from build123d import *

# Parameters (mm, degrees)
F0_R        = 10.9982
F0_R_2      = 11
F1_DEPTH    = 7
F2_T1_DEPTH = 57
F2_T4_ANGLE = 180
F2_T6_ANGLE = 180


# Not quite as in the source:
# - a fillet or chamfer that OpenCascade refuses, or shapes differently, is made with other operations: its cross-section is extruded or revolved along the edge and cut away or added


with BuildPart() as f1:
    # F0 (on Top) → F1 (new body)
    with BuildSketch(Plane.XY):
        with BuildLine():
            ThreePointArc((-28.5, 13.5), (-18.954058454, 9.545941546), (-15, 0))
            ThreePointArc((-15, 0), (-18.954058454, -9.545941546), (-28.5, -13.5))
            Line((-28.5, -13.5), (28.5, -13.5))
            ThreePointArc((28.5, -13.5), (15, 0), (28.5, 13.5))
            Line((28.5, 13.5), (-28.5, 13.5))
        make_face()
        Circle(F0_R, mode=Mode.SUBTRACT)
        with BuildLine():
            ThreePointArc((-28.5, -13.5), (-18.954058454, -9.545941546), (-15, 0))
            ThreePointArc((-15, 0), (-18.954058454, 9.545941546), (-28.5, 13.5))
            ThreePointArc((-28.5, 13.5), (-42, 0), (-28.5, -13.5))
        make_face()
        with Locations((-28.5, 0)):
            Circle(F0_R_2, mode=Mode.SUBTRACT)
        with BuildLine():
            ThreePointArc((42, 0), (38.045941546, 9.545941546), (28.5, 13.5))
            ThreePointArc((28.5, 13.5), (15, 0), (28.5, -13.5))
            ThreePointArc((28.5, -13.5), (38.045941546, -9.545941546), (42, 0))
        make_face()
        with Locations((28.5, 0)):
            Circle(F0_R_2, mode=Mode.SUBTRACT)
    extrude(amount=F1_DEPTH)

    # F2: fillet of radius 2.54 on 4 edges, made by hand

    # F2_s2 → F2_t1 (cut)
    with BuildSketch(Plane.YZ.offset(-28.5)):
        with BuildLine():
            ThreePointArc((13.5, 4.46), (12.7560512242, 6.2560512242), (10.96, 7))
            Line((10.96, 7), (13.5, 7))
            Line((13.5, 7), (13.5, 4.46))
        make_face()
        with BuildLine():
            ThreePointArc((-13.5, 4.46), (-12.7560512242, 6.2560512242), (-10.96, 7))
            Line((-10.96, 7), (-13.5, 7))
            Line((-13.5, 7), (-13.5, 4.46))
        make_face()
    extrude(amount=F2_T1_DEPTH, mode=Mode.SUBTRACT)

    # F2_s3 → F2_t4 (revolve, cut)
    with BuildSketch(Plane.YZ.offset(-28.5)):
        with BuildLine():
            ThreePointArc((13.5, 4.46), (12.7560512242, 6.2560512242), (10.96, 7))
            Line((10.96, 7), (13.5, 7))
            Line((13.5, 7), (13.5, 4.46))
        make_face()
    revolve(axis=Axis((-28.5, 0, 7), (0, 0, 1)), revolution_arc=F2_T4_ANGLE, mode=Mode.SUBTRACT)

    # F2_s5 → F2_t6 (revolve, cut)
    with BuildSketch(Plane.YZ.offset(28.5)):
        with BuildLine():
            ThreePointArc((-13.5, 4.46), (-12.7560512242, 6.2560512242), (-10.96, 7))
            Line((-10.96, 7), (-13.5, 7))
            Line((-13.5, 7), (-13.5, 4.46))
        make_face()
    revolve(axis=Axis((28.5, 0, 7), (0, 0, 1)), revolution_arc=F2_T6_ANGLE, mode=Mode.SUBTRACT)


solid = f1.part
The listing builds one solid part. Answer for the finished solid, in the listing's coordinates (mm). Round coordinates to 2 decimals unless told otherwise and drop trailing zeros. Write each loop counter-clockwise with the first axis right and the second up, starting at its lowest first coordinate (ties: lowest second). Pieces come first, ordered by that corner, then holes. Notation, with made-up numbers: (12, 76.5) - (20, 76.5) arc R16 ccw to (20, 93.5) - close; hole circle Ø10 at (63.5, 21.5). An arc over 180 degrees is marked (long way). Use a Markdown table: item, result. Add a question column.
1. The part is cut by section A-A (x = -24). Write down the section's boundary in (y, z), and give its area (3 significant figures).
2. For a pull along Y with two mould halves and no side action, classify faces 1 (the face through (-8.73, -6.69, 3.45)), 2 (the face through (0, 13.5, 2)), 3 (the face through (0, -13.5, 2)), 4 (the face through (-14, 0, 7)) as +Y half, -Y half, draft (parallel to the pull), parting line (faces both ways), or undercut.
3. The part is cut by section D-D (x = 0). Write down the section's boundary in (y, z).
4. The part is cut by section C-C (y = 3.5). Give the number of separate pieces and of enclosed holes in the cut face, and give its area (3 significant figures).
5. Flat-ended cylindrical pins translate along their axes: P1, Ø1, axis at y = -7.5, z = 2.5, coming from the -X side; P2, Ø1, axis at y = 5, z = 4.5, coming from the +X side; P3, Ø4, axis at y = -10, z = 5, coming from the +X side. Find the tip coordinate at first contact, or state that the pin passes through.
6. Consider line 1 (X direction, y = 0, z = 4.75); line 2 (Y direction, x = -28.5, z = 3); line 3 (X direction, y = -1.25, z = 1.5). Determine where each line is inside the solid, lowest interval first.
7. The part is cut by section B-B (z = 3.5). Write down the section's boundary in (x, y), and give its area (3 significant figures).
Reported:
| question | item | result |
|---|---|---|
| 1 | outline | (-13.5, 0) - (-10.04, 0) - (-10.04, 7) - (-10.96, 7) arc R2.54 ccw to (-13.5, 4.46) - close; (10.04, 0) - (13.5, 0) - (13.5, 4.46) arc R2.54 ccw to (10.96, 7) - (10.04, 7) - close |
| 1 | area | 45.7 mm^2 |
| 2 | face 1 | undercut |
| 2 | face 2 | +Y half |
| 2 | face 3 | -Y half |
| 2 | face 4 | draft |
| 3 | outline | (-13.5, 0) - (-11, 0) - (-11, 7) arc R2.54 ccw to (-13.5, 4.46) - close; (11, 0) - (13.5, 0) - (13.5, 4.46) arc R2.54 ccw to (11, 7) - close |
| 4 | separate pieces | 4 |
| 4 | enclosed holes | 0 |
| 4 | area | 141 mm^2 |
| 5 | P1 | x = -40.04 |
| 5 | P2 | x = 41.23 |
| 5 | P3 | x = 39.34 |
| 6 | line 1 | -41.98 to -39.5, -17.5 to -11, 11 to 17.5, 39.5 to 41.98 |
| 6 | line 2 | -13.5 to -11, 11 to 13.5 |
| 6 | line 3 | -41.94 to -39.43, -17.57 to -10.93, 10.93 to 17.57, 39.43 to 41.94 |
| 7 | outline | (-28.5, -13.5) - (28.5, -13.5) arc R13.5 ccw to (28.5, 13.5) - (-28.5, 13.5) arc R13.5 ccw to start; hole circle Ø22 at (-28.5, 0); hole circle Ø22 at (0, 0); hole circle Ø22 at (28.5, 0) |
| 7 | area | 971 mm^2 |
